Can you work these out from the model? Positions are in its coordinate system, mm. Give positions to 0.01 mm unless a question says otherwise; leave off trailing zeros. Loops run counter-clockwise (first coordinate to the right, second up) from the corner with the lowest first, then second, coordinate; pieces in that order, holes last. Notation, with made-up numbers: (16.25, -0.5) - (30.25, -0.5) arc R16 cw to (30.25, 29.5) - close; hole circle Ø1 at (88, 59.5). An arc over 180 degrees is marked (long way). Answer in a Markdown table with one row per item.
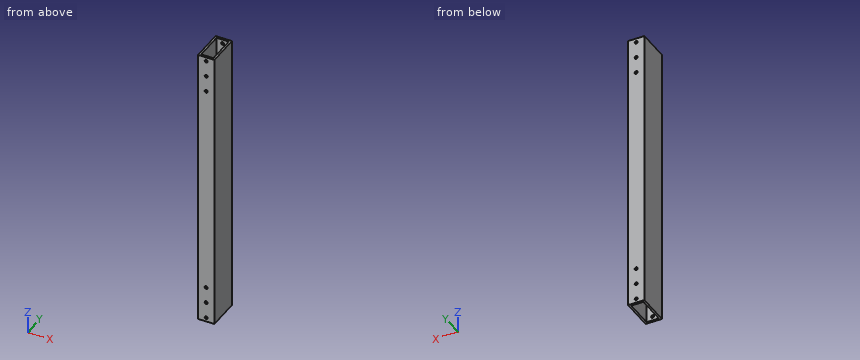
from build123d import *

# Parameters (mm, degrees)
SKETCH1_W           = 25.4
SKETCH1_H           = 50.8
BOSS_EXTRUDE1_DEPTH = 444.5
SHELL1_T            = -3.175
SKETCH2_R           = 2.38125
CUT_EXTRUDE1_DEPTH  = 448.573658742


with BuildPart() as part:
    # Sketch1 → Boss-Extrude1 (new body)
    with BuildSketch(Plane.XY):
        Rectangle(SKETCH1_W, SKETCH1_H)
    extrude(amount=BOSS_EXTRUDE1_DEPTH)

    # Shell1
    shell1_openings = [part.faces().sort_by_distance(p)[0] for p in [
        (0, 0, 444.5),
        (0, 0, 0),
    ]]
    offset(amount=SHELL1_T, openings=shell1_openings, kind=Kind.INTERSECTION)

    # Sketch2 → Cut-Extrude1 (cut, through all)
    with BuildSketch(Plane(origin=(0, 25.4, 0), x_dir=(1, 0, 0), z_dir=(0, 1, 0))):
        with Locations(Location((0, -6.35, 0), (0, 0, 270))):
            Circle(SKETCH2_R)
        with Locations(Location((0, -31.75, 0), (0, 0, 270))):
            Circle(SKETCH2_R)
        with Locations(Location((0, -57.15, 0), (0, 0, 270))):
            Circle(SKETCH2_R)
        with Locations(Location((0, -387.35, 0), (0, 0, 270))):
            Circle(SKETCH2_R)
        with Locations(Location((0, -412.75, 0), (0, 0, 270))):
            Circle(SKETCH2_R)
        with Locations(Location((0, -438.15, 0), (0, 0, 270))):
            Circle(SKETCH2_R)
    extrude(amount=-CUT_EXTRUDE1_DEPTH, mode=Mode.SUBTRACT)


solid = part.part
Q1. If I drill on line 1 (X direction, y = 12, z = 426) (3 decimals); line 2 (Y direction, x = -2.5, z = 81) (3 decimals); line 3 (X direction, y = -23, z = 57), over which ranges is the centre line in solid material (lowest first)? Write a range as [from, to].
Checked values:
| item | result |
|---|---|
| line 1 | x = [-12.7, -9.525], [9.525, 12.7] |
| line 2 | y = [-25.4, -22.225], [22.225, 25.4] |
| line 3 | x = [-12.7, -2.38], [2.38, 12.7] |
Q2. For pin 1 (4.5 mm diameter, centred on x = 0, z = 6.35, fed in from +Y), with a flat end and sliding along its axis, tell me the tip position at first contact or that it passes through.
Checked values:
| item | result |
|---|---|
| pin 1 | passes through |
Q3. Imagine slicing it at A-A, the plane y = -11.5. Write out the boundary of the cut face in (x, z) (3 decimals), and give its area (3 significant figures).
Checked values:
| item | result |
|---|---|
| outline | (-12.7, 0) - (-9.525, 0) - (-9.525, 444.5) - (-12.7, 444.5) - close; (9.525, 0) - (12.7, 0) - (12.7, 444.5) - (9.525, 444.5) - close |
| area | 2,820 mm² |
